The figure shows three views and two pictorial views of one solid part (mm, origin at its lowest corner). Answer the questions. A direction names the side the tool comes from. Give positions to 0.01 mm unless a question says otherwise; leave off trailing zeros. Order: outer loops, then holes, each group sorted by start corner. A loop starts at its lowest first (then second) coordinate and runs counter-clockwise, first axis right, second up. Notation, with made-up numbers: M 86.5,-14 L 96.5,-14 A25 cw 96.5,14 Z; hole C 46,8.5 d5. An arc over 180 degrees is marked long. Write item = value, one per line. Start each with the question number.
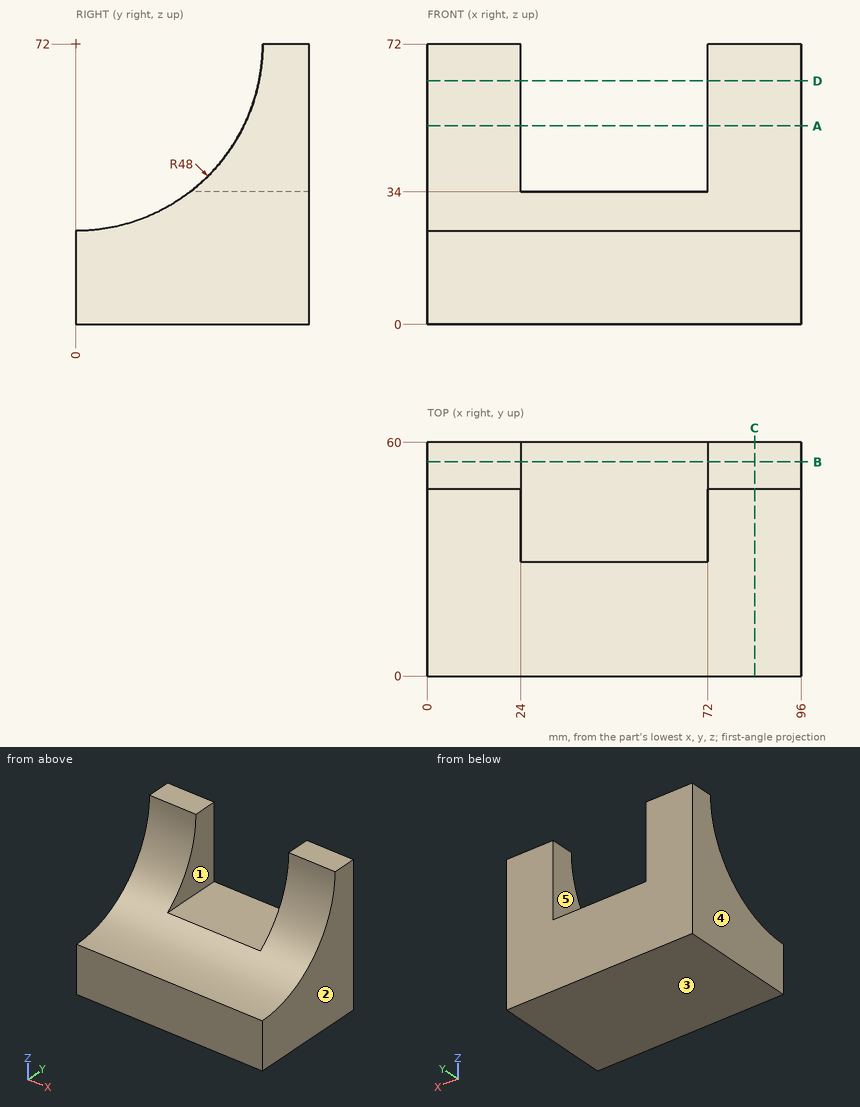
1) For the marked faces 1 and 2, determine the directions among +Z, -Z, +X, -X, +Y, -Y from which every point of the face is accessible in a straight line to the end or side of a thin tool.
2) Find section D-D on z = 62.5. Determine the outline of the cut face in (x, y), plus the area to 3 significant figures.
3) For a pull along X with two mould halves and no side action, classify the marked faces 3, 4 and 5 as pulls with the +X half, pulls with the -X half, needs draft (parallel to the pull), parting line crosses it, or undercut.
4) Find section A-A on z = 51. Determine the outline of the cut face in (x, y), plus the area to 3 significant figures.
5) This flat-tipped pin is pushed along its axis until it touches: P1, Ø12, axis at x = 33, y = 51, coming from the +Z side. Where does it stop, or does it pass through?
6) Find section C-C on x = 84. Determine the outline of the cut face in (y, z), plus the area to 3 significant figures.
7) Find the intervals of material crossed by probe 1 along X at (y, z) = (50.5, 40); probe 2 along Z at (x, y) = (60, 57); probe 3 along Z at (x, y) = (77, 44), in increasing order. Write a range as [from, to].
8) Find section B-B on y = 55. Determine the outline of the cut face in (x, z), plus the area to 3 significant figures.
Numbers:
q1.face_1 = +Z, +Y, -Y
q1.face_2 = +Z, -Z, +X, +Y, -Y
q2.outline = M 0,47.05 L 24,47.05 L 24,60 L 0,60 Z; M 72,47.05 L 96,47.05 L 96,60 L 72,60 Z
q2.area = 622 mm2
q3.face_3 = needs draft
q3.face_4 = pulls with the -X half
q3.face_5 = undercut
q4.outline = M 0,43.16 L 24,43.16 L 24,60 L 0,60 Z; M 72,43.16 L 96,43.16 L 96,60 L 72,60 Z
q4.area = 808 mm2
q5.P1 = 34
q6.outline = M 0,0 L 60,0 L 60,72 L 48,72 A48 cw 0,24 Z
q6.area = 2,510 mm2
q7.probe_1 = [0, 24], [72, 96]
q7.probe_2 = [0, 34]
q7.probe_3 = [0, 52.82]
q8.outline = M 0,0 L 96,0 L 96,72 L 72,72 L 72,34 L 24,34 L 24,72 L 0,72 Z
q8.area = 5,090 mm2
